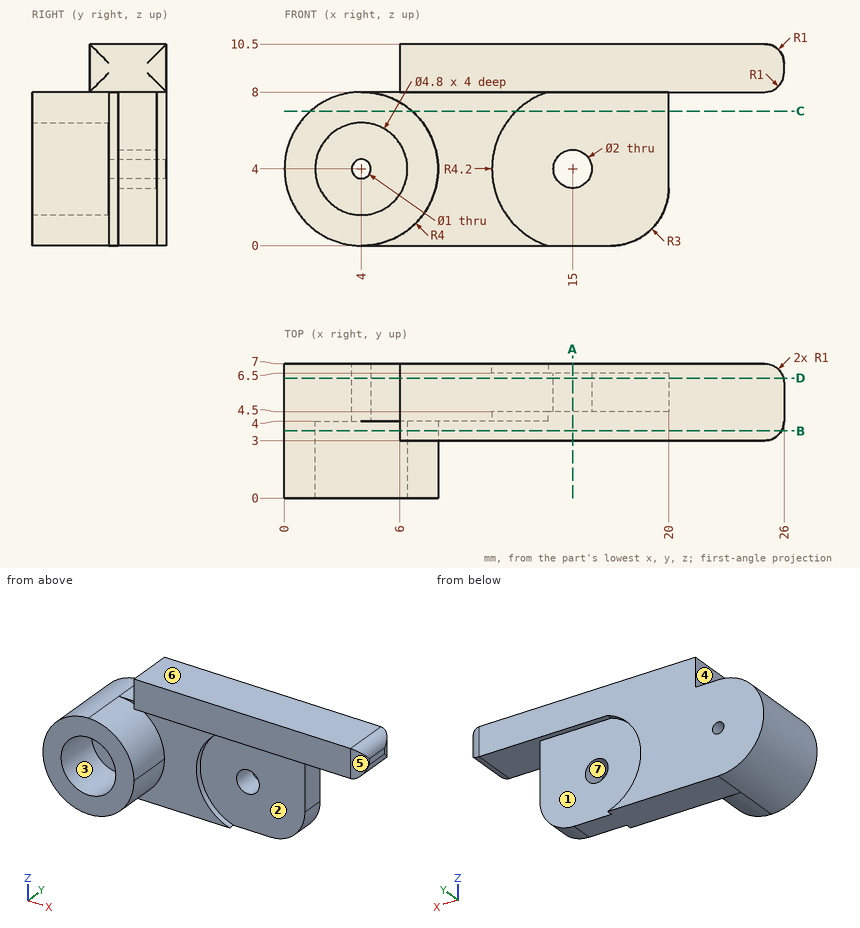
Print and shaded views of the part. All mm, measured from the part's lowest x, y and z. A direction names the side the tool comes from. Coordinates: 2 decimals unless noted, no trailing zeros. Order: outer loops, then holes, each group sorted by start corner. A loop starts at its lowest first (then second) coordinate and runs counter-clockwise, first axis right, second up.
(1) Pull direction X, two halves, no side cores. Call the marked faces 5, 6 and 7: pulls with the +X half, pulls with the -X half, needs draft (parallel to the pull), parting line crosses it, or undercut.
Check sheet entries:
face 5: pulls with the +X half
face 6: needs draft
face 7: undercut
(2) Slice it at B-B, the plane y = 3.5. Write the cut outline in (x, z), and give its area (3 significant figures).
Check sheet entries:
outline: circle Ø8 at (4, 4); (6, 8) - (25, 8) arc R1 ccw to (25.87, 8.5) - (25.87, 10) arc R1 ccw to (25, 10.5) - (6, 10.5) - close; hole circle Ø4.8 at (4, 4)
area: 81.6 mm2
(3) Slice it at D-D, the plane y = 6.25. Write the cut outline in (x, z).
Check sheet entries:
outline: (4, 0) - (17, 0) arc R3 ccw to (20, 3) - (20, 8) - (25, 8) arc R1 ccw to (25.97, 8.75) - (25.97, 9.75) arc R1 ccw to (25, 10.5) - (6, 10.5) - (6, 8) - (4, 8) arc R4 ccw to start; hole circle Ø1 at (4, 4); hole circle Ø2 at (15, 4)
(4) Probe L1, parallel to Z at x = 4, y = 2.85; L2, parallel to Z at x = 15, y = 5.1; L3, parallel to Y at x = 6.5, z = 7.5. List the from-to ranges inside material, lowest first.
Check sheet entries:
L1: z = 0 to 1.6, 6.4 to 8
L2: z = 0 to 3, 5 to 10.5
L3: y = 4 to 7
(5) Slice it at C-C, the plane z = 7. Write the cut outline in (x, y).
Check sheet entries:
outline: (1.35, 0) - (6.65, 0) - (6.65, 4) - (12.06, 4) - (12.06, 4.5) - (20, 4.5) - (20, 6.5) - (12.06, 6.5) - (12.06, 7) - (1.35, 7) - close
(6) Slice it at A-A, the plane x = 15. Write the cut outline in (y, z).
Check sheet entries:
outline: (3, 8) - (4.5, 8) - (4.5, 5) - (6.5, 5) - (6.5, 8) - (7, 8) - (7, 10.5) - (3, 10.5) - close; (4.5, 0) - (6.5, 0) - (6.5, 3) - (4.5, 3) - close
(7) Tool access for the marked faces 1, 2, 3 and 4: list every direction of +Z, -Z, +X, -X, +Y, -Y with a clear straight run to the whole face (end or side of a thin tool).
Check sheet entries:
face 1: +X, +Y
face 2: +X, -Y
face 3: -Y
face 4: +Z, -X, +Y, -Y
(8) Pin check, flat tips, straight feed: pin 1 Ø1.5 at (x, z) = (5.5, 1) entering from -Y; pin 2 Ø1.4 at (x, z) = (3, 4.5) entering from -Y; pin 3 Ø1.5 at (x, z) = (17, 4) entering from +Y; pin 4 Ø2 at (y, z) = (5.5, 9.5) entering from -X. Stop position of each tip, or through.
Check sheet entries:
pin 1: stops at y = 0
pin 2: stops at y = 4
pin 3: stops at y = 6.5
pin 4: stops at x = 6
